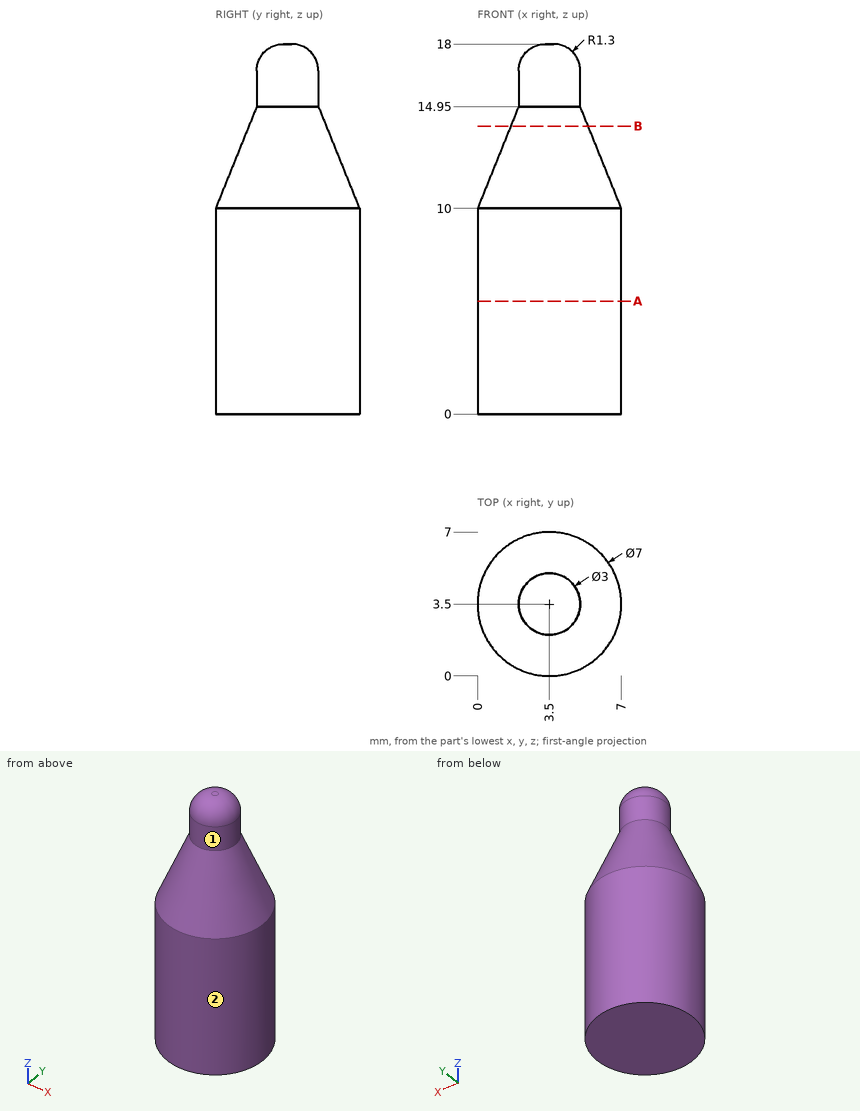
Answer from the drawing. Dimensions are ordinates in mm from the lowest x, y and z of the part. A direction names the side the tool comes from. Round coordinates to 2 decimals unless told otherwise and drop trailing zeros. Loops run counter-clockwise (first coordinate to the right, second up) from the corner with the lowest first, then second, coordinate; pieces in that order, holes last.
(1) For the marked faces 1 and 2, determine the directions among +Z, -Z, +X, -X, +Y, -Y from which every point of the face is accessible in a straight line to the end or side of a thin tool.
Computed values:
face 1: +Z
face 2: +Z, -Z
(2) Find the intervals of material crossed by L1, parallel to Y at x = 3, z = 11.75; L2, parallel to X at y = 4, z = 8; L3, parallel to Z at x = 4.75, y = 6 (1 decimal), in increasing order.
Computed values:
L1: y = 0.75 to 6.25
L2: x = 0.04 to 6.96
L3: z = 0 to 11.7
(3) Each of these flat-tipped pins is pushed along its axis until it touches: P1, Ø1.5, axis at x = 2.5, y = 6, coming from the +Z side (1 decimal); P2, Ø2, axis at y = 2.5, z = 16, coming from the +X side. Where does it stop, or does it pass through?
Computed values:
P1: stops at z = 13.9
P2: stops at x = 5
(4) The part is cut by section B-B, the plane z = 14. Give the vertices of the cut face in (x, y), and give its area (4 significant figures).
Computed values:
outline: circle Ø3.77 at (3.5, 3.5)
area: 11.15 mm2
(5) The part is cut by section A-A, the plane z = 5.5. Give the vertices of the cut face in (x, y).
Computed values:
outline: circle Ø7 at (3.5, 3.5)
